Model file for the job. Use its own axes, mm. Coordinates: 2 decimals unless noted, no trailing zeros. Loops run counter-clockwise (first coordinate to the right, second up) from the corner with the lowest first, then second, coordinate; pieces in that order, holes last.
from build123d import *

# Parameters (mm, degrees)
BOSS_EXTRUDE1_DEPTH   = 10
SKETCH2_W             = 162
SKETCH2_H             = 20
CUT_EXTRUDE1_DEPTH    = 0.5
CUT_EXTRUDE2_DEPTH    = 67.5
F_6_0MM_DOWEL_HOLE2_D = 5.9
F_6_0MM_DOWEL_HOLE4_D = 5.9
SKETCH30_R            = 1.65
CUT_EXTRUDE7_DEPTH    = 20
SKETCH31_W            = 11.000242512
SKETCH31_H            = 20
BOSS_EXTRUDE2_DEPTH   = 0.5
SKETCH5_R             = 1.7
CUT_EXTRUDE3_DEPTH    = 115


with BuildPart() as part:
    # Sketch1 → Boss-Extrude1 (new body, symmetric)
    with BuildSketch(Plane(origin=(0, 0, 0), x_dir=(1, 0, 0), z_dir=(0, 1, 0))):
        with BuildLine():
            Line((0, 70), (0, 81))
            ThreePointArc((0, 81), (-81, 0), (0, -81))
            Line((0, -81), (0, -70))
            ThreePointArc((0, -70), (-70, 0), (0, 70))
        make_face()
    extrude(amount=BOSS_EXTRUDE1_DEPTH, both=True)

    # Sketch2 → Cut-Extrude1 (cut)
    with BuildSketch(Plane(origin=(0, 0, 0), x_dir=(0, 0, -1), z_dir=(1, 0, 0))):
        Rectangle(SKETCH2_W, SKETCH2_H)
    extrude(amount=-CUT_EXTRUDE1_DEPTH, mode=Mode.SUBTRACT)

    # Sketch4 → Cut-Extrude2 (cut)
    with BuildSketch(Plane(origin=(-75, 0, 0), x_dir=(0, 0, -1), z_dir=(1, 0, 0))):
        Polygon((-72.117199752, 2.825), (-75.379228773, 2.825), (-77.010243284, 0), (-75.379228773, -2.825), (-72.117199752, -2.825), (-70.486185242, 0), align=None)
        Polygon((80.510485796, 0), (78.879471286, 2.825), (75.617442265, 2.825), (73.986427755, 0), (75.617442265, -2.825), (78.879471286, -2.825), align=None)
    extrude(amount=CUT_EXTRUDE2_DEPTH, mode=Mode.SUBTRACT)

    # Ø6.0mm Dowel Hole2 (through all)
    with Locations(Plane(origin=(0, 0, 0), x_dir=(-0.707106781, 0, -0.707106781), z_dir=(0.707106781, 0, -0.707106781))):
        with Locations((0, 0)):
            Hole(F_6_0MM_DOWEL_HOLE2_D / 2)

    # Ø6.0mm Dowel Hole4 (through all)
    with Locations(Plane(origin=(0, 0, 0), x_dir=(0.707106781, 0, -0.707106781), z_dir=(0.707106781, 0, 0.707106781))):
        with Locations((0, 0)):
            Hole(F_6_0MM_DOWEL_HOLE4_D / 2)

    # Sketch30 → Cut-Extrude7 (cut, symmetric)
    with BuildSketch(Plane.XZ.offset(10)):
        with Locations((-41.894091711, 62.810310298)):
            Circle(SKETCH30_R)
        with Locations((-71.513705419, 24.208261757)):
            Circle(SKETCH30_R)
    extrude(amount=CUT_EXTRUDE7_DEPTH, both=True, mode=Mode.SUBTRACT)

    # Sketch31 → Boss-Extrude2 (add)
    with BuildSketch(Plane(origin=(-0.5, 0, 0), x_dir=(0, 0, -1), z_dir=(1, 0, 0))):
        with Locations((-75.498335519, 0)):
            Rectangle(SKETCH31_W, SKETCH31_H)
        with Locations((75.498335519, 0)):
            Rectangle(SKETCH31_W, SKETCH31_H)
    extrude(amount=BOSS_EXTRUDE2_DEPTH)

    # Sketch5 → Cut-Extrude3 (cut, symmetric)
    with BuildSketch(Plane(origin=(-75, 0, 0), x_dir=(0, 0, -1), z_dir=(1, 0, 0))):
        with Locations((77.248456775, 0)):
            Circle(SKETCH5_R)
        with Locations((-73.748214263, 0)):
            Circle(SKETCH5_R)
    extrude(amount=CUT_EXTRUDE3_DEPTH, both=True, mode=Mode.SUBTRACT)


solid = part.part
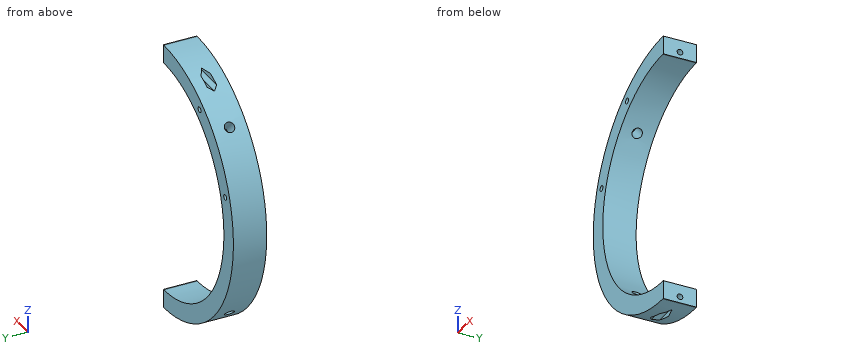
Q1. Slice it at A-A (x = -10.5). List the corners of the cut face in (y, z) (3 decimals).
Answers:
outline: (-10, -80.317) - (-0.336, -80.317) - (-2.825, -78.879) - (-2.825, -75.617) - (0, -73.986) - (2.825, -75.617) - (2.825, -78.879) - (0.336, -80.317) - (10, -80.317) - (10, -69.208) - (-10, -69.208) - close; (-10, 69.208) - (10, 69.208) - (10, 80.317) - (-10, 80.317) - close; hole (-2.825, 72.117) - (0, 70.486) - (2.825, 72.117) - (2.825, 75.379) - (0, 77.01) - (-2.825, 75.379) - close
Q2. Flat gauge pins, fed straight in: P1, Ø1.5, axis at y = -4.5, z = -24.5, coming from the +X side; P2, Ø3, axis at y = 0, z = -77.25, coming from the -X side; P3, Ø3, axis at y = 0.5, z = 73.5, coming from the -X side; P4, Ø5, axis at x = -44, y = 3.5, coming from the -Z side. Where does each tip first touch, or does it go through?
Answers:
P1: stops at x = -65.29
P2: passes through
P3: stops at x = -7.5
P4: stops at z = -69.56
Q3. Slice it at B-B (y = 5). List the corners of the cut face in (x, z), and give its area (3 significant figures).
Answers:
outline: (-0.5, -81) - (0, -81) - (0, -70) - (-0.5, -70) arc R70 cw to (-0.5, 70) - (0, 70) - (0, 81) - (-0.5, 81) arc R81 ccw to start; hole circle Ø3.3 at (-71.51, 24.21); hole circle Ø3.3 at (-41.89, 62.81)
area: 2,590 mm2
Q4. Slice it at C-C (x = -27). List the corners of the cut face in (y, z) (3 decimals).
Answers:
outline: (-10, -76.368) - (-2.825, -76.368) - (-2.825, -75.617) - (0, -73.986) - (2.825, -75.617) - (2.825, -76.368) - (10, -76.368) - (10, -64.583) - (-10, -64.583) - close; (-10, 64.583) - (10, 64.583) - (10, 76.368) - (1.113, 76.368) - (2.825, 75.379) - (2.825, 72.117) - (0, 70.486) - (-2.825, 72.117) - (-2.825, 75.379) - (-1.113, 76.368) - (-10, 76.368) - close
Q5. Drill centre lines: line 1 (Z direction, x = -6, y = -3.75); line 2 (Z direction, x = -34.5, y = -7.25); line 3 (X direction, y = -6.75, z = 70.5). Where is each one in solid material? Low to high.
Answers:
line 1: z = -80.78 to -69.74, 69.74 to 80.78
line 2: z = -73.29 to -60.91, 60.91 to 73.29
line 3: x = -39.88 to 0
Q6. Slice it at D-D (z = 0). List the corners of the cut face in (x, y), and give its area (3 significant figures).
Answers:
outline: (-81, -10) - (-70, -10) - (-70, 10) - (-81, 10) - close
area: 220 mm2
